```python
from build123d import *

# Parameters (mm, degrees)
SKETCH1_W           = 11.865
SKETCH1_H           = 10.16
SKETCH1_W_2         = 28.77
SKETCH1_H_2         = 23.06
BOSS_EXTRUDE1_DEPTH = 9
SKETCH3_R           = 7.65
CUT_EXTRUDE1_DEPTH  = 36.220996579


with BuildPart() as part:
    # Sketch1 → Boss-Extrude1 (new body)
    with BuildSketch(Plane.XY):
        with Locations((-20.3175, 6.45)):
            Rectangle(SKETCH1_W, SKETCH1_H)
        with Locations((0, -10.16)):
            Rectangle(SKETCH1_W_2, SKETCH1_H_2)
        with Locations((0, 6.45)):
            Rectangle(SKETCH1_W_2, SKETCH1_H)
        with Locations((0, 16.61)):
            Rectangle(SKETCH1_W_2, SKETCH1_H)
        with Locations((20.3175, 6.45)):
            Rectangle(SKETCH1_W, SKETCH1_H)
    extrude(amount=BOSS_EXTRUDE1_DEPTH)

    # Sketch3 → Cut-Extrude1 (cut, through all)
    with BuildSketch(Plane.XY.offset(9)):
        with Locations((0, 6.35)):
            Circle(SKETCH3_R)
    extrude(amount=-CUT_EXTRUDE1_DEPTH, mode=Mode.SUBTRACT)


solid = part.part
```
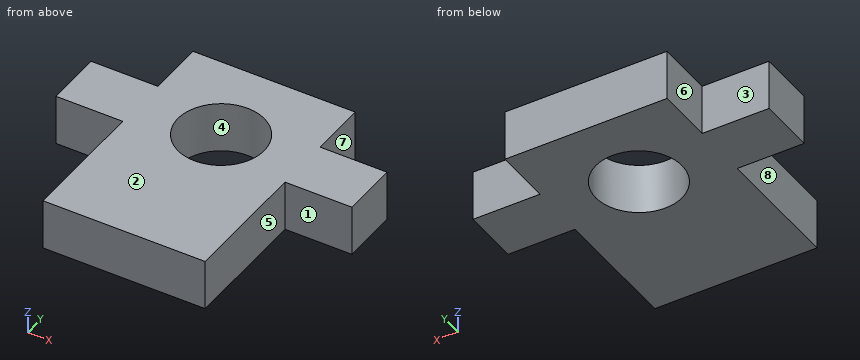
Check sheet for the modelled part. Datum: model origin and axes. Units: mm. Face numbers are marked on the shaded views. A direction names the side the tool comes from. Round coordinates to 2 decimals unless told otherwise and drop trailing zeros. Loops run counter-clockwise (first coordinate to the right, second up) from the corner with the lowest first, then second, coordinate; pieces in that order, holes last. Notation, with made-up numbers: (-15.5, -28) -> (38.5, -28) arc R28 cw to (38.5, 7) -> close; hole circle Ø8 at (-7, 52). An arc over 180 degrees is marked (long way). Write item = value, one per line. Start each with the question number.
1) Release check for a two-part mould opening along Y. For the marked faces 1, 2, 3 and 4 record: released by +Y, released by -Y, zero draft, split by the parting line, or undercut.
2) Gauge pin test, flat ends, axial feed: pin 1 Ø2.5 at (y, z) = (-8.5, 4) entering from -X (3 decimals); pin 2 Ø2.5 at (x, z) = (-20, 6) entering from +Y; pin 3 Ø14 at (x, y) = (0, 6.35) entering from +Z; pin 4 Ø4.5 at (y, z) = (18.5, 5.5) entering from +X (3 decimals). Record the tip position at first contact, or that the pin passes through.
3) Sectioned sample at B-B, the plane y = 6.35. Record the cut outline in (x, z), plus the area to 3 significant figures.
4) Sectioned sample at A-A, the plane x = 0. Record the cut outline in (y, z).
5) Sectioned sample at C-C, the plane z = 6.5. Record the cut outline in (x, y) (3 decimals), plus the area to 3 significant figures.
6) Set-up check for the marked faces 5, 6, 7 and 8: record each of +Z, -Z, +X, -X, +Y, -Y from which the full face is reachable in a straight line by a thin tool's end or side.
7) Thickness scan on probe 1 along Y at (x, z) = (0, 3); probe 2 along X at (y, z) = (-9, 2) (3 decimals); probe 3 along X at (y, z) = (10, 3.75). Record the ranges inside material, lowest first.
8) Sectioned sample at D-D, the plane x = 18.5. Record the cut outline in (y, z), plus the area to 3 significant figures.
Results are:
q1.face_1 = released by -Y
q1.face_2 = zero draft
q1.face_3 = released by +Y
q1.face_4 = undercut
q2.pin_1 = -14.385
q2.pin_2 = 11.53
q2.pin_3 = through
q2.pin_4 = 14.385
q3.outline = (-26.25, 0) -> (-7.65, 0) -> (-7.65, 9) -> (-26.25, 9) -> close; (7.65, 0) -> (26.25, 0) -> (26.25, 9) -> (7.65, 9) -> close
q3.area = 335 mm^2
q4.outline = (-21.69, 0) -> (-1.3, 0) -> (-1.3, 9) -> (-21.69, 9) -> close; (14, 0) -> (21.69, 0) -> (21.69, 9) -> (14, 9) -> close
q5.outline = (-26.25, 1.37) -> (-14.385, 1.37) -> (-14.385, -21.69) -> (14.385, -21.69) -> (14.385, 1.37) -> (26.25, 1.37) -> (26.25, 11.53) -> (14.385, 11.53) -> (14.385, 21.69) -> (-14.385, 21.69) -> (-14.385, 11.53) -> (-26.25, 11.53) -> close; hole circle Ø15.3 at (0, 6.35)
q5.area = 1,310 mm^2
q6.face_5 = +Z, -Z, +X, -Y
q6.face_6 = +Z, -Z, -X, +Y
q6.face_7 = +Z, -Z, +X, +Y
q6.face_8 = +Z, -Z, -X, -Y
q7.probe_1 = -21.69 to -1.3, 14 to 21.69
q7.probe_2 = -14.385 to 14.385
q7.probe_3 = -26.25 to -6.72, 6.72 to 26.25
q8.outline = (1.37, 0) -> (11.53, 0) -> (11.53, 9) -> (1.37, 9) -> close
q8.area = 91.4 mm^2
